Geometry: final body of the model. Coordinates: model frame, mm. Face numbers are marked on the shaded views. A direction names the side the tool comes from. Give positions to 0.01 mm unless a question says otherwise; leave off trailing zeros. Order: outer loops, then holes, each group sorted by start corner. A loop starts at its lowest first (then second) coordinate and runs counter-clockwise, first axis right, second up. Notation, with made-up numbers: M 50,-35 L 80,-35 A12 ccw 80,-18 Z; hole C -21,-24 d2. An arc over 180 degrees is marked long. Use CSV: the item, a comma, the result in double quotes.
```python
from build123d import *

# Parameters (mm, degrees)
F0_W     = 20
F0_H     = 20
F1_DEPTH = 3
F2_W     = 2
F2_H     = 20
F3_DEPTH = 27
F5_DEPTH = 25
F6_R     = 1.5
F7_DEPTH = 25
F8_R     = 3


with BuildPart() as f1:
    # F0 (on Front) → F1 (new body)
    with BuildSketch(Plane.XZ):
        with Locations((10, -10)):
            Rectangle(F0_W, F0_H)
    extrude(amount=F1_DEPTH)

    # F2 (on face) → F3 (join)
    with BuildSketch(Plane(origin=(0, 0, 0), x_dir=(-1, 0, 0), z_dir=(0, 1, 0))):
        with Locations((-1, -10)):
            Rectangle(F2_W, F2_H)
    extrude(amount=F3_DEPTH)

    # F4 (on face) → F5 (cut)
    with BuildSketch(Plane.XZ.offset(3)):
        with BuildLine():
            Line((5.8, -5.006674), (5.8, -10.993326))
            ThreePointArc((5.8, -10.993326), (11, -14), (16.2, -10.993326))
            Line((16.2, -10.993326), (16.2, -5.006674))
            ThreePointArc((16.2, -5.006674), (11, -2), (5.8, -5.006674))
        make_face()
    extrude(amount=-F5_DEPTH, mode=Mode.SUBTRACT)

    # F6 (on face) → F7 (cut)
    with BuildSketch(Plane.YZ.offset(2)):
        with Locations((12, -10)):
            Circle(F6_R)
    extrude(amount=-F7_DEPTH, mode=Mode.SUBTRACT)

    # F8
    f8_edges = [f1.edges().sort_by_distance(p)[0] for p in [
        (20, -1.5, 0),
    ]]
    fillet(f8_edges, radius=F8_R)


solid = f1.part
```
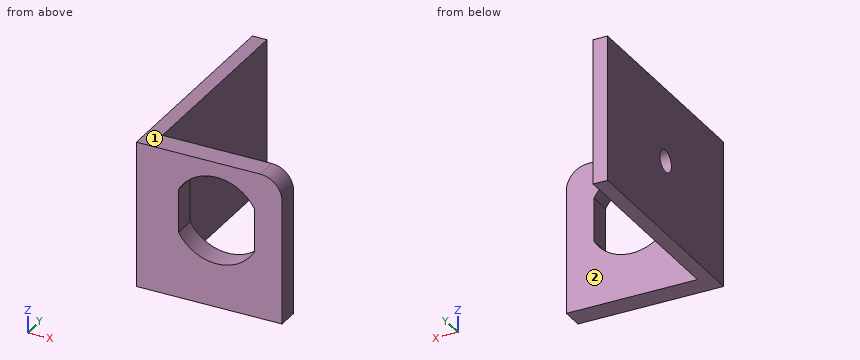
1. Reachability of the marked faces 1 and 2 from +Z, -Z, +X, -X, +Y, -Y: full face, straight path, thin tool, end or side. Return the list, or none.
Answer:
face 1,"+Z, +X, -X, +Y, -Y"
face 2,"+Z, -Z, +X, +Y"
2. Section D-D, the plane y = -0.5. Return the cut outline in (x, z), plus the area to 3 significant figures.
Answer:
outline,"M 0,-20 L 20,-20 L 20,-3 A3 ccw 17,0 L 0,0 Z; hole M 5.8,-10.99 A6 ccw 16.2,-10.99 L 16.2,-5.01 A6 ccw 5.8,-5.01 Z"
area,"291 mm2"
3. Section C-C, the plane z = -10. Return the cut outline in (x, y).
Answer:
outline,"M 0,-3 L 5.8,-3 L 5.8,0 L 2,0 L 2,10.5 L 0,10.5 Z; M 0,13.5 L 2,13.5 L 2,27 L 0,27 Z; M 16.2,-3 L 20,-3 L 20,0 L 16.2,0 Z"
4. Section B-B, the plane x = 11. Return the cut outline in (y, z), plus the area to 3 significant figures.
Answer:
outline,"M -3,-20 L 0,-20 L 0,-14 L -3,-14 Z; M -3,-2 L 0,-2 L 0,0 L -3,0 Z"
area,"24.0 mm2"
5. Section A-A, the plane y = 12. Return the cut outline in (x, z).
Answer:
outline,"M 0,-20 L 2,-20 L 2,-11.5 L 0,-11.5 Z; M 0,-8.5 L 2,-8.5 L 2,0 L 0,0 Z"
6. Pin query (flat end, axial travel): pin 1 Ø10 at (x, z) = (13, -2) entering from +Y; pin 2 Ø3 at (y, z) = (8.5, -10) entering from +X. Return the tip coordinate at first contact, or that it passes through.
Answer:
pin 1,"y = 0"
pin 2,"x = 2"
7. Line query: line 1 (Z direction, x = 1.65, y = 12); line 2 (X direction, y = -0.5, z = -7); line 3 (X direction, y = 13.5, z = -17.5). Output: solid intervals per line, ascending.
Answer:
line 1,"-20 to -11.5, -8.5 to 0"
line 2,"0 to 5.8, 16.2 to 20"
line 3,"0 to 2"
